Input: part model. Units: mm. Frame: model coordinates. Face numbers are marked on the shaded views. A direction names the side the tool comes from. Coordinates: 2 decimals unless noted, no trailing zeros. Write each loop counter-clockwise with the first axis right and the second up, starting at its lowest first coordinate (ties: lowest second). Pieces come first, ordered by that corner, then holes. Notation, with made-up numbers: M 79,51 L 98,51 A36 cw 98,88 Z; hole C 69.25,1 d8. An arc over 180 degrees is marked long. Write each question's results on one line, items separated by ' | '. Start each with the question number.
1. First-contact query: pin 1 (1 mm diameter, centred on y = 1.5, z = -1, fed in from +X); pin 2 (0.6 mm diameter, centred on y = 0.5, z = -0.5, fed in from -X). Flat tips, straight axial feed; report the tip coordinate or a pass-through.
2. Ray query, probe 1 along Z at (x, y) = (2.25, 1.8); probe 2 along X at (y, z) = (0.1, 1.5); probe 3 along Z at (x, y) = (5, 0.1). Return the intervals inside material, ascending.
3. Section query A-A, the plane x = 0. Output: boundary loops of the cut face in (y, z), and give its area (3 significant figures).
4. Set-up query: the marked faces 5, 6 and 7. Return all of +Z, -Z, +X, -X, +Y, -Y with unobstructed straight access to the full face (end or side cutting, diameter ignored); none if empty.
5. Section query D-D, the plane x = -6. Output: boundary loops of the cut face in (y, z), and give its area (3 significant figures).
6. Section query C-C, the plane z = -1.75. Output: boundary loops of the cut face in (x, y).
7. Section query B-B, the plane y = 0.45. Output: boundary loops of the cut face in (x, z).
8. Pull-direction query (Z, two-part tool) for the marked faces 1, 2, 3 and 4; classes: +Z half, -Z half, draft (parallel to the pull), parting line (faces both ways), or undercut.
```python
from build123d import *

# Parameters (mm, degrees)
SKETCH1_W           = 9
SKETCH1_H           = 8
SKETCH1_W_2         = 6
SKETCH1_H_2         = 5
BOSS_EXTRUDE1_DEPTH = 2
SKETCH2_W           = 15
SKETCH2_H           = 3.2
BOSS_EXTRUDE3_DEPTH = 2


with BuildPart() as part:
    # Sketch1 → Boss-Extrude1 (new body)
    with BuildSketch(Plane(origin=(0, 0, 0), x_dir=(1, 0, 0), z_dir=(0, 1, 0))):
        Rectangle(SKETCH1_W, SKETCH1_H)
        Rectangle(SKETCH1_W_2, SKETCH1_H_2, mode=Mode.SUBTRACT)
    extrude(amount=BOSS_EXTRUDE1_DEPTH)

    # Sketch2 → Boss-Extrude3 (add)
    with BuildSketch(Plane(origin=(0, 0, 0), x_dir=(1, 0, 0), z_dir=(0, 1, 0))):
        with Locations((0, -5.6)):
            Rectangle(SKETCH2_W, SKETCH2_H)
    extrude(amount=BOSS_EXTRUDE3_DEPTH)


solid = part.part
```
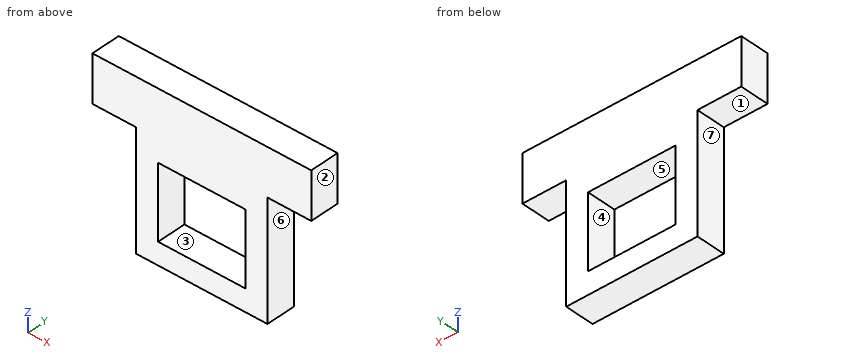
Answer:
1) pin 1: x = 4.5 | pin 2: x = -4.5
2) probe 1: -4 to -2.5, 2.5 to 7.2 | probe 2: -4.5 to -3, 3 to 4.5 | probe 3: 4 to 7.2
3) outline: M 0,-4 L 2,-4 L 2,-2.5 L 0,-2.5 Z; M 0,2.5 L 2,2.5 L 2,7.2 L 0,7.2 Z | area: 12.4 mm^2
4) face 5: +Y, -Y | face 6: -Z, +X, +Y, -Y | face 7: -Z, -X, +Y, -Y
5) outline: M 0,4 L 2,4 L 2,7.2 L 0,7.2 Z | area: 6.40 mm^2
6) outline: M -4.5,0 L -3,0 L -3,2 L -4.5,2 Z; M 3,0 L 4.5,0 L 4.5,2 L 3,2 Z
7) outline: M -7.5,4 L -4.5,4 L -4.5,-4 L 4.5,-4 L 4.5,4 L 7.5,4 L 7.5,7.2 L -7.5,7.2 Z; hole M -3,-2.5 L 3,-2.5 L 3,2.5 L -3,2.5 Z
8) face 1: -Z half | face 2: draft | face 3: undercut | face 4: undercut
